Input: part model. Units: mm. Frame: model coordinates. A direction names the side the tool comes from. Round coordinates to 2 decimals unless told otherwise and drop trailing zeros. Loops run counter-clockwise (first coordinate to the right, second up) from the corner with the lowest first, then second, coordinate; pieces in that order, holes last. Notation, with made-up numbers: (23, -40) -> (32, -40) arc R18 ccw to (32, -18) -> close; hole circle Ø11 at (59, 49.25). An arc over 180 degrees is marked (long way). Answer in a Markdown table with one row per item. Add a question column.
Q1. Reachability of faces 4 (the face through (-5.25, 2, 2)), 5 (the face through (-10, 10, 2)), 6 (the face through (0, -5.75, 2)) from +Z, -Z, +X, -X, +Y, -Y: full face, straight path, thin tool, end or side. Return the list, or none.
Q2. Mould query, pull axis X, two halves, no side actions, for faces 1 (the face through (5, 12, 2)), 2 (the face through (-5, 12, 2)), 3 (the face through (-5.125, -7, 2)). Classes: pulls with the +X half, pulls with the -X half, needs draft (parallel to the pull), parting line crosses it, or undercut.
Q3. Section C-C, the plane y = 3.75. Output: boundary loops of the cut face in (x, z), and give its area (3 significant figures).
Q4. Section B-B, the plane z = 3.65. Output: boundary loops of the cut face in (x, y) (3 decimals).
Q5. Pin query (flat end, axial travel): pin 1 (1.2 mm diameter, centred on x = 1.5, z = 2, fed in from -Y); pin 2 (2 mm diameter, centred on x = -12, z = 2.5, fed in from +Y); pin 3 (3 mm diameter, centred on x = -10, y = -1.5, fed in from -Z). Return the tip coordinate at first contact, or that it passes through.
Q6. Section D-D, the plane x = 13. Output: boundary loops of the cut face in (y, z).
Q7. Ray query, L1, parallel to X at y = 3.75, z = 0.9; L2, parallel to Y at x = 3.5, z = 2.9; L3, parallel to X at y = -7.5, z = 0.45 (3 decimals). Return the intervals inside material, ascending. Write a range as from..to.
Q8. Section A-A, the plane x = -2.25. Output: boundary loops of the cut face in (y, z), and give its area (3 significant figures).
```python
from build123d import *

# Parameters (mm, degrees)
SKETCH_W  = 10.5
SKETCH_H  = 4.25
PAD_DEPTH = 4
FILLET_R  = 1


with BuildPart() as part:
    # Sketch → Pad (new body)
    with BuildSketch(Plane.XY):
        Polygon((-15, 10), (-15, -10), (-5.125, -10), (-5.125, -5.75), (5.125, -5.75), (5.125, -10), (15, -10), (15, 10), (5, 10), (5, 14), (-5, 14), (-5, 10), align=None)
        with Locations((0, 2.125)):
            Rectangle(SKETCH_W, SKETCH_H, mode=Mode.SUBTRACT)
    extrude(amount=PAD_DEPTH)

    # Fillet
    fillet_edges = [part.edges().sort_by_distance(p)[0] for p in [
        (-5.125, -10, 2),
        (5.125, -10, 2),
    ]]
    fillet(fillet_edges, radius=FILLET_R)


solid = part.part
```
Answer block:
| question | item | result |
|---|---|---|
| 1 | face 4 | +Z, -Z |
| 1 | face 5 | +Z, -Z, -X, +Y |
| 1 | face 6 | +Z, -Z, -Y |
| 2 | face 1 | pulls with the +X half |
| 2 | face 2 | pulls with the -X half |
| 2 | face 3 | undercut |
| 3 | outline | (-15, 0) -> (-5.25, 0) -> (-5.25, 4) -> (-15, 4) -> close; (5.25, 0) -> (15, 0) -> (15, 4) -> (5.25, 4) -> close |
| 3 | area | 78.0 mm^2 |
| 4 | outline | (-15, -10) -> (-6.125, -10) arc R1 ccw to (-5.125, -9) -> (-5.125, -5.75) -> (5.125, -5.75) -> (5.125, -9) arc R1 ccw to (6.125, -10) -> (15, -10) -> (15, 10) -> (5, 10) -> (5, 14) -> (-5, 14) -> (-5, 10) -> (-15, 10) -> close; hole (-5.25, 0) -> (5.25, 0) -> (5.25, 4.25) -> (-5.25, 4.25) -> close |
| 5 | pin 1 | y = -5.75 |
| 5 | pin 2 | y = 10 |
| 5 | pin 3 | z = 0 |
| 6 | outline | (-10, 0) -> (10, 0) -> (10, 4) -> (-10, 4) -> close |
| 7 | L1 | -15..-5.25, 5.25..15 |
| 7 | L2 | -5.75..0, 4.25..14 |
| 7 | L3 | -15..-5.125, 5.125..15 |
| 8 | outline | (-5.75, 0) -> (0, 0) -> (0, 4) -> (-5.75, 4) -> close; (4.25, 0) -> (14, 0) -> (14, 4) -> (4.25, 4) -> close |
| 8 | area | 62.0 mm^2 |
